```python
from build123d import *

# Parameters (mm, degrees)
F1_DEPTH = 88.9
F2_R     = 11.212602
F3_DEPTH = 76.2
F4_R     = 10.819094
F5_DEPTH = 76.2


with BuildPart() as f1:
    # F0 (on Right) → F1 (new body)
    with BuildSketch(Plane.YZ):
        Polygon((63.066408, -39.499849), (63.066408, 39.499849), (23.723558, 39.499849), (23.723558, 0), (-30.519336, 0), (-30.519336, 39.499849), (-63.066408, 39.499849), (-63.066408, -39.499849), align=None)
    extrude(amount=F1_DEPTH)

    # F2 (on Front) → F3 (cut)
    with BuildSketch(Plane.XZ):
        with Locations((41.055754, 15.218571)):
            Circle(F2_R)
    extrude(amount=F3_DEPTH, mode=Mode.SUBTRACT)

    # F4 (on Front) → F5 (cut)
    with BuildSketch(Plane.XZ):
        with Locations((46.320774, 13.538517)):
            Circle(F4_R)
    extrude(amount=-F5_DEPTH, mode=Mode.SUBTRACT)


solid = f1.part
```
Input: part model. Units: mm. Frame: model coordinates. A direction names the side the tool comes from. Round coordinates to 2 decimals unless told otherwise and drop trailing zeros. Loops run counter-clockwise (first coordinate to the right, second up) from the corner with the lowest first, then second, coordinate; pieces in that order, holes last. Notation, with made-up numbers: M 57,58 L 80,58 A11 ccw 80,71 Z; hole C 21.25,56.25 d6. An arc over 180 degrees is marked long. Answer in a Markdown table with one row per item. Add a question column.
1. Section B-B (z = 11.5). Output: boundary loops of the cut face in (x, y).
2. Section C-C (x = 12). Output: boundary loops of the cut face in (y, z).
3. Mould query, pull axis Y, two halves, no side actions, for faces 5 (the face through (44, -30.519, 28)), 6 (the face through (44, 44, 39.5)), 7 (the face through (44, 63.066, -1)). Classes: released by +Y, released by -Y, zero draft, split by the parting line, or undercut.
4. Ray query, probe 1 along Y at (x, z) = (22, 31); probe 2 along Y at (x, z) = (55, 18); probe 3 along Z at (x, y) = (74, 2). Return the intervals inside material, ascending.
5. Set-up query: faces 1 (the face through (51.75, -46.57, 18.59)), 2 (the face through (43.8, 23.724, 24.4)), 3 (the face through (35.51, 43.12, 14.01)), 4 (the face through (88.9, -1, -8)). Return all of +Z, -Z, +X, -X, +Y, -Y with unobstructed straight access to the full face (end or side cutting, diameter ignored); none if empty.
6. Section A-A (x = 43.5). Output: boundary loops of the cut face in (y, z).
7. Section D-D (y = -22). Output: boundary loops of the cut face in (x, z), and give its area (3 significant figures).
Values follow:
| question | item | result |
|---|---|---|
| 1 | outline | M 0,-63.07 L 30.48,-63.07 L 30.48,-30.52 L 0,-30.52 Z; M 0,23.72 L 35.7,23.72 L 35.7,63.07 L 0,63.07 Z; M 51.63,-63.07 L 88.9,-63.07 L 88.9,-30.52 L 51.63,-30.52 Z; M 56.95,23.72 L 88.9,23.72 L 88.9,63.07 L 56.95,63.07 Z |
| 2 | outline | M -63.07,-39.5 L 63.07,-39.5 L 63.07,39.5 L 23.72,39.5 L 23.72,0 L -30.52,0 L -30.52,39.5 L -63.07,39.5 Z |
| 3 | face 5 | undercut |
| 3 | face 6 | zero draft |
| 3 | face 7 | released by +Y |
| 4 | probe 1 | -63.07 to -30.52, 23.72 to 63.07 |
| 4 | probe 2 | -63.07 to -30.52 |
| 4 | probe 3 | -39.5 to 0 |
| 5 | face 1 | -Y |
| 5 | face 2 | +Z, +X, -X |
| 5 | face 3 | +Y |
| 5 | face 4 | +Z, -Z, +X, +Y, -Y |
| 6 | outline | M -63.07,-39.5 L 63.07,-39.5 L 63.07,3.09 L 23.72,3.09 L 23.72,0 L -30.52,0 L -30.52,4.28 L -63.07,4.28 Z; M -63.07,26.16 L -30.52,26.16 L -30.52,39.5 L -63.07,39.5 Z; M 23.72,23.98 L 63.07,23.98 L 63.07,39.5 L 23.72,39.5 Z |
| 7 | outline | M 0,-39.5 L 88.9,-39.5 L 88.9,0 L 0,0 Z |
| 7 | area | 3,510 mm^2 |
